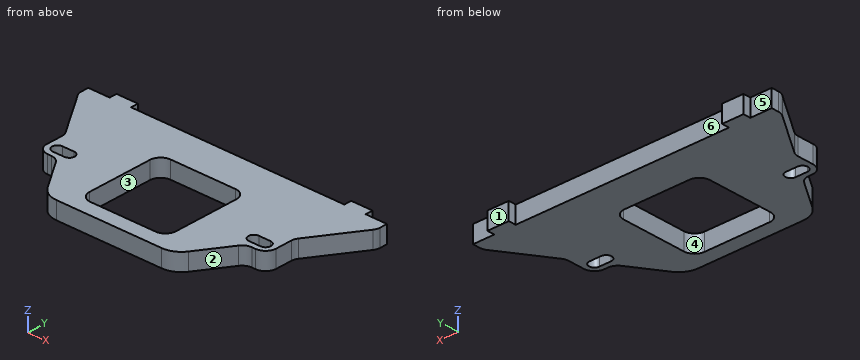
```python
from build123d import *

# Parameters (mm, degrees)
SKETCH_1_W          = 81
SKETCH_1_H          = 81
EXTRUDE_1_DEPTH     = 8
FILLET_1_R          = 10
CUT_EXTRUDE_1_DEPTH = 16
FILLET_2_R          = 20
FILLET_3_R          = 10


with BuildPart() as part:
    # 草图1 → 凸台-拉伸1 (new, symmetric)
    with BuildSketch(Plane.XY):
        Polygon((60, 0), (-60, 0), (-88.666666667, 43), (-107.5, 43), (-107.5, 71.25), (-140, 120), (-140, 130), (-120, 130), (-120, 137), (-100, 137), (-100, 130), (100, 130), (100, 137), (120, 137), (120, 130), (140, 130), (140, 120), (107.5, 71.25), (107.5, 43), (88.666666667, 43), align=None)
        with Locations((0, 54.5)):
            Rectangle(SKETCH_1_W, SKETCH_1_H, mode=Mode.SUBTRACT)
    extrude(amount=EXTRUDE_1_DEPTH, both=True)

    # 圆角1
    fillet_1_edges = [part.edges().sort_by_distance(p)[0] for p in [
        (-107.5, 43, 0),
        (107.5, 43, 0),
        (40.5, 14, 0),
        (40.5, 95, 0),
        (-40.5, 95, 0),
        (-40.5, 14, 0),
    ]]
    fillet(fillet_1_edges, radius=FILLET_1_R)

    # 草图2 → 切除-拉伸1 (cut)
    with BuildSketch(Plane.XY.offset(8)):
        with BuildLine():
            Line((-97.5, 58), (-86.5, 58))
            ThreePointArc((-86.5, 58), (-81.5, 53), (-86.5, 48))
            Line((-86.5, 48), (-97.5, 48))
            ThreePointArc((-97.5, 48), (-102.5, 53), (-97.5, 58))
        make_face()
        with BuildLine():
            Line((97.5, 48), (86.5, 48))
            ThreePointArc((86.5, 48), (81.5, 53), (86.5, 58))
            Line((86.5, 58), (97.5, 58))
            ThreePointArc((97.5, 58), (102.5, 53), (97.5, 48))
        make_face()
    extrude(amount=-CUT_EXTRUDE_1_DEPTH, mode=Mode.SUBTRACT)

    # 圆角2
    fillet_2_edges = [part.edges().sort_by_distance(p)[0] for p in [
        (60, 0, 0),
        (-60, 0, 0),
    ]]
    fillet(fillet_2_edges, radius=FILLET_2_R)

    # 圆角3
    fillet_3_edges = [part.edges().sort_by_distance(p)[0] for p in [
        (-88.666666667, 43, 0),
        (-107.5, 71.25, 0),
        (-140, 120, 0),
        (140, 120, 0),
        (107.5, 71.25, 0),
        (88.666666667, 43, 0),
    ]]
    fillet(fillet_3_edges, radius=FILLET_3_R)


solid = part.part
```
Can you work these out from the model? Positions are in its coordinate system, mm. Face numbers are marked on the shaded views. A direction names the side the tool comes from. Give positions to 0.01 mm unless a question says otherwise; leave off trailing zeros. Loops run counter-clockwise (first coordinate to the right, second up) from the corner with the lowest first, then second, coordinate; pieces in that order, holes last. Notation, with made-up numbers: M 37.25,29 L 55.25,29 A14 cw 55.25,52 Z; hole C -15,38 d3. An arc over 180 degrees is marked long. One line per item, written item: value.
(1) Will these pins go through, and if not, where does the flat tip stop? pin 1 (3.5 mm diameter, centred on y = 132, z = 1, fed in from -X); pin 2 (9 mm diameter, centred on x = -89.5, z = 3, fed in from +Y); pin 3 (4.5 mm diameter, centred on y = 62, z = -4, fed in from -X); pin 4 (1.5 mm diameter, centred on x = -16.5, z = 4, fed in from -Y).
Returned:
pin 1: x = -120
pin 2: y = 130
pin 3: x = -107.5
pin 4: y = 0
(2) Suppose I cut it at A-A on x = -12.5. List the corners of the cut face in (y, z) for me, plus the area to 3 significant figures.
Returned:
outline: M 0,-8 L 14,-8 L 14,8 L 0,8 Z; M 95,-8 L 130,-8 L 130,8 L 95,8 Z
area: 784 mm^2
(3) I need wall thicknesses on line 1 (Y direction, x = -28.5, z = -2); line 2 (Y direction, x = -31.5, z = -2.5); line 3 (X direction, y = 67.5, z = -1). Which ranges of each line are inside material? Lowest first, please.
Returned:
line 1: 0 to 14, 95 to 130
line 2: 0 to 14.05, 94.95 to 130
line 3: -107.5 to -40.5, 40.5 to 107.5
(4) We'd pull the mould along X, two halves only. Please class the marked faces 1, 2 and 3: released by +X, released by -X, zero draft, split by the parting line, or undercut.
Returned:
face 1: zero draft
face 2: released by +X
face 3: undercut
(5) Suppose I cut it at C-C on z = 2.75. Count the separate pieces of the cut face and the enclosed holes in it, plus the area to 3 significant figures.
Returned:
separate pieces: 1
enclosed holes: 3
area: 20,700 mm^2
(6) Which directions (+Z, -Z, +X, -X, +Y, -Y) give clear straight access to the entire face, cutting with the end or side of a thin tool? Please do the marked faces 4, 5 and 6.
Returned:
face 4: +Z, -Z
face 5: +Z, -Z, -X, +Y
face 6: +Z, -Z, +Y
(7) Suppose I cut it at B-B on y = 31. List the corners of the cut face in (x, z) for me, plus the area to 3 significant figures.
Returned:
outline: M -80.67,-8 L -40.5,-8 L -40.5,8 L -80.67,8 Z; M 40.5,-8 L 80.67,-8 L 80.67,8 L 40.5,8 Z
area: 1,290 mm^2
(8) Suppose I cut it at D-D on y = 104. List the corners of the cut face in (x, z) for me.
Returned:
outline: M -129.33,-8 L 129.33,-8 L 129.33,8 L -129.33,8 Z
